from build123d import *

# Parameters (mm, degrees)
SKETCH1_W           = 176
SKETCH1_H           = 166
BOSS_EXTRUDE1_DEPTH = 128
SKETCH3_W           = 30
SKETCH3_H           = 15
CUT_EXTRUDE1_DEPTH  = 15
FILLET1_R           = 2.54
SKETCH4_W           = 12
SKETCH4_H           = 12
SKETCH4_R           = 2.75
BOSS_EXTRUDE2_DEPTH = 2


with BuildPart() as part:
    # Sketch1 → Boss-Extrude1 (new body)
    with BuildSketch(Plane(origin=(0, 0, 0), x_dir=(1, 0, 0), z_dir=(0, 1, 0))):
        with Locations((0, 83)):
            Rectangle(SKETCH1_W, SKETCH1_H)
    extrude(amount=BOSS_EXTRUDE1_DEPTH)

    # Sketch3 → Cut-Extrude1 (cut)
    with BuildSketch(Plane(origin=(0, 128, 0), x_dir=(1, 0, 0), z_dir=(0, 1, 0))):
        with Locations((73, 7.5)):
            Rectangle(SKETCH3_W, SKETCH3_H)
    cut_extrude1 = extrude(amount=-CUT_EXTRUDE1_DEPTH, mode=Mode.SUBTRACT)

    # Fillet1
    fillet1_edges = [part.edges().sort_by_distance(p)[0] for p in [
        (88, 56.5, 0),
        (0, 0, -166),
        (88, 0, -83),
        (0, 0, 0),
        (-88, 0, -83),
        (-88, 64, -166),
        (88, 64, -166),
        (-88, 64, 0),
    ]]
    fillet(fillet1_edges, radius=FILLET1_R)

    # Sketch4 → Boss-Extrude2 (add)
    with BuildSketch(Plane(origin=(80.38, 0, 0), x_dir=(0, 0, -1), z_dir=(1, 0, 0))):
        with Locations((7.5, 119)):
            Rectangle(SKETCH4_W, SKETCH4_H)
        with Locations((7.5, 120)):
            Circle(SKETCH4_R, mode=Mode.SUBTRACT)
    boss_extrude2 = extrude(amount=-BOSS_EXTRUDE2_DEPTH)

    # Mirror2: Cut-Extrude1, Boss-Extrude2 across plane
    add(cut_extrude1.mirror(Plane(origin=(0, 0, 0), x_dir=(0, 0, 1), z_dir=(1, 0, 0))), mode=Mode.SUBTRACT)
    add(boss_extrude2.mirror(Plane(origin=(0, 0, 0), x_dir=(0, 0, 1), z_dir=(1, 0, 0))))


solid = part.part
Could you check a few things on this model? Use its own coordinates, in mm. A direction names the side the tool comes from. Give positions to 0.01 mm unless a question says otherwise; leave off trailing zeros. Order: outer loops, then holes, each group sorted by start corner. A loop starts at its lowest first (then second) coordinate and runs counter-clockwise, first axis right, second up.
1. For faces 4 (the cylindrical face through (79.394, 117.315, -6.904)), 5 (the flat face through (-80.38, 116, -7)), 6 (the flat face through (88, 64, -82)), 7 (the flat face through (80.38, 116, -7)), 8 (the flat face through (-58, 121, -7)), which set-ups out of +Z, -Z, +X, -X, +Y, -Y let a thin tool reach every point of the face, with its end or its side?
2. Suppose I cut it at A-A (z = -7.5). List the corners of the cut face in (x, y) for me.
3. We'd pull the mould along Y, two halves only. Please class faces 1 (the flat face through (-1, 0, -84)), 2 (the cylindrical face through (-79.394, 117.315, -6.904)), 3 (the flat face through (-1, 64, 0)): pulls with the +Y half, pulls with the -Y half, needs draft (parallel to the pull), parting line crosses it, or undercut.
4. Suppose I cut it at B-B (y = 120). List the corners of the cut face in (x, z) for me, plus the area to 3 significant figures.
5. Will these pins go through, and if not, where does the flat tip stop? P1, Ø16.5, axis at x = -67.5, y = 121.5, coming from the +Z side; P2, Ø4.5, axis at y = 120, z = -7.5, coming from the -X side; P3, Ø6, axis at y = 117.5, z = -6.5, coming from the -X side.
6. I need wall thicknesses on L1, parallel to Y at x = -78.9, z = -7.5; L2, parallel to Y at x = 78, z = -7. Which ranges of each line are inside material? Lowest first, please.
Solved:
1. face 4: +X
1. face 5: +Z, -X, +Y
1. face 6: +Z, -Z, +X, +Y, -Y
1. face 7: +Z, +X, +Y
1. face 8: +Z, +Y
2. outline: (-88, 2.54) arc R2.54 ccw to (-85.46, 0) - (85.46, 0) arc R2.54 ccw to (88, 2.54) - (88, 113) - (80.38, 113) - (80.38, 117.25) - (78.38, 117.25) - (78.38, 113) - (58, 113) - (58, 128) - (-58, 128) - (-58, 113) - (-78.38, 113) - (-78.38, 117.25) - (-80.38, 117.25) - (-80.38, 113) - (-88, 113) - close; (-80.38, 122.75) - (-78.38, 122.75) - (-78.38, 125) - (-80.38, 125) - close; (78.38, 122.75) - (80.38, 122.75) - (80.38, 125) - (78.38, 125) - close
3. face 1: pulls with the -Y half
3. face 2: undercut
3. face 3: needs draft
4. outline: (-88, -163.46) arc R2.54 ccw to (-85.46, -166) - (85.46, -166) arc R2.54 ccw to (88, -163.46) - (88, -15) - (58, -15) - (58, 0) - (-58, 0) - (-58, -15) - (-88, -15) - close; (-80.38, -13.5) - (-78.38, -13.5) - (-78.38, -10.25) - (-80.38, -10.25) - close; (-80.38, -4.75) - (-78.38, -4.75) - (-78.38, -1.5) - (-80.38, -1.5) - close; (78.38, -13.5) - (80.38, -13.5) - (80.38, -10.25) - (78.38, -10.25) - close; (78.38, -4.75) - (80.38, -4.75) - (80.38, -1.5) - (78.38, -1.5) - close
4. area: 28,300 mm2
5. P1: stops at z = -15
5. P2: stops at x = -58
5. P3: stops at x = -80.38
6. L1: y = 0 to 117.25, 122.75 to 125
6. L2: y = 0 to 113
